from build123d import *

# Parameters (mm, degrees)
BOSS_EXTRUDE1_DEPTH = 6
SKETCH3_R           = 2
CUT_EXTRUDE1_DEPTH  = 2.5
CUT_EXTRUDE5_REACH  = 11.713
SKETCH5_R           = 2
SKETCH6_R           = 2
BOSS_EXTRUDE2_DEPTH = 1
CUT_EXTRUDE6_REACH  = 12.36
SKETCH7_R           = 4


with BuildPart() as part:
    # Sketch2 → Boss-Extrude1 (new body)
    with BuildSketch(Plane.XY):
        Polygon((0, -5.773502692), (5, -2.886751346), (5, 2.886751346), (0, 5.773502692), (-5, 2.886751346), (-5, -2.886751346), align=None)
    extrude(amount=BOSS_EXTRUDE1_DEPTH)

    # Sketch3 → Cut-Extrude1 (cut)
    with BuildSketch(Plane.ZY.offset(5)):
        with Locations(Location((3, 0, 0), (0, 0, 270))):
            Circle(SKETCH3_R)
    extrude(amount=-CUT_EXTRUDE1_DEPTH, mode=Mode.SUBTRACT)

    # Sketch5 → Cut-Extrude5 (cut, up to next)
    with BuildSketch(Plane.XY.offset(6), mode=Mode.PRIVATE) as cut_extrude5_sk1:
        Circle(SKETCH5_R)
    cut_extrude5_tool1 = extrude(cut_extrude5_sk1.sketch, amount=-CUT_EXTRUDE5_REACH, mode=Mode.PRIVATE) & part.part
    add(cut_extrude5_tool1.solids().sort_by_distance((0, 0, 6))[0], mode=Mode.SUBTRACT)

    # Sketch6 → Boss-Extrude2 (add)
    with BuildSketch(Plane(origin=(0, 0, 0), x_dir=(-1, 0, 0), z_dir=(0, 0, -1))):
        Polygon((0, 5.773502692), (-5, 2.886751346), (-5, -2.886751346), (0, -5.773502692), (5, -2.886751346), (5, 2.886751346), align=None)
        with Locations(Location((0, 0, 0), (0, 0, 180))):
            Circle(SKETCH6_R, mode=Mode.SUBTRACT)
    extrude(amount=BOSS_EXTRUDE2_DEPTH)

    # Sketch7 → Cut-Extrude6 (cut, up to next)
    with BuildSketch(Plane(origin=(0, 0, -1), x_dir=(-1, 0, 0), z_dir=(0, 0, -1)), mode=Mode.PRIVATE) as cut_extrude6_sk1:
        Circle(SKETCH7_R)
    cut_extrude6_tool1 = extrude(cut_extrude6_sk1.sketch, amount=-CUT_EXTRUDE6_REACH, mode=Mode.PRIVATE) & part.part
    add(cut_extrude6_tool1.solids().sort_by_distance((0, 0, -1))[0], mode=Mode.SUBTRACT)


solid = part.part
Geometry check sheet. Reference: the model listing, model coordinates, mm. Give positions to 0.01 mm unless a question says otherwise; leave off trailing zeros. Write each loop counter-clockwise with the first axis right and the second up, starting at its lowest first coordinate (ties: lowest second). Pieces come first, ordered by that corner, then holes. Notation, with made-up numbers: (6.5, 0.25) - (54.5, 0.25) arc R5 cw to (54.5, 6.25) - close; hole circle Ø8 at (64.5, 41). An arc over 180 degrees is marked (long way). Put each result on its own line as item: value.
1. Go/stop test with a flat-tipped pin: pin 1 (3.5 mm diameter, centred on y = 0, z = 3, fed in from -X). Record where the tip stops, or that it passes through.
Ans:
pin 1: stops at x = 3.6
2. Sectioned sample at B-B, the plane y = 3.25. Enter the section's corners in (x, z).
Ans:
outline: (-4.37, -1) - (-2.33, -1) - (-2.33, 6) - (-4.37, 6) - close; (2.33, -1) - (4.37, -1) - (4.37, 6) - (2.33, 6) - close
3. Draft check along Y on faces 1 (the flat face through (-2.465, -4.35, 2.549)), 2 (the cylindrical face through (-4.413, -1.847, 2.234)), 3 (the flat face through (-3, -3, 6)). Enter one of: +Y half, -Y half, draft (parallel to the pull), parting line (faces both ways), or undercut.
Ans:
face 1: -Y half
face 2: undercut
face 3: draft
4. Sectioned sample at A-A, the plane x = -2.75. Enter the section's corners in (y, z).
Ans:
outline: (-4.19, -1) - (-2.9, -1) - (-2.9, 6) - (-4.19, 6) - close; (2.9, -1) - (4.19, -1) - (4.19, 6) - (2.9, 6) - close
5. Sectioned sample at C-C, the plane z = 5.5. Enter the section's corners in (x, y), plus the area to 3 significant figures.
Ans:
outline: (-5, -2.89) - (0, -5.77) - (5, -2.89) - (5, 2.89) - (0, 5.77) - (-5, 2.89) - close; hole circle Ø8 at (0, 0)
area: 36.3 mm²
6. Thickness scan on line 1 (Z direction, x = -4.55, y = 0); line 2 (Y direction, x = -0.25, z = 0.25); line 3 (X direction, y = -2.75, z = 3.25). Record the ranges inside material, lowest first.
Ans:
line 1: z = -1 to 1, 5 to 6
line 2: y = -5.63 to -3.99, 3.99 to 5.63
line 3: x = -5 to -2.9, 2.9 to 5
7. Sectioned sample at D-D, the plane y = 0. Enter the section's corners in (x, z).
Ans:
outline: (-5, -1) - (-4, -1) - (-4, 1) - (-5, 1) - close; (-5, 5) - (-4, 5) - (-4, 6) - (-5, 6) - close; (4, -1) - (5, -1) - (5, 6) - (4, 6) - close
